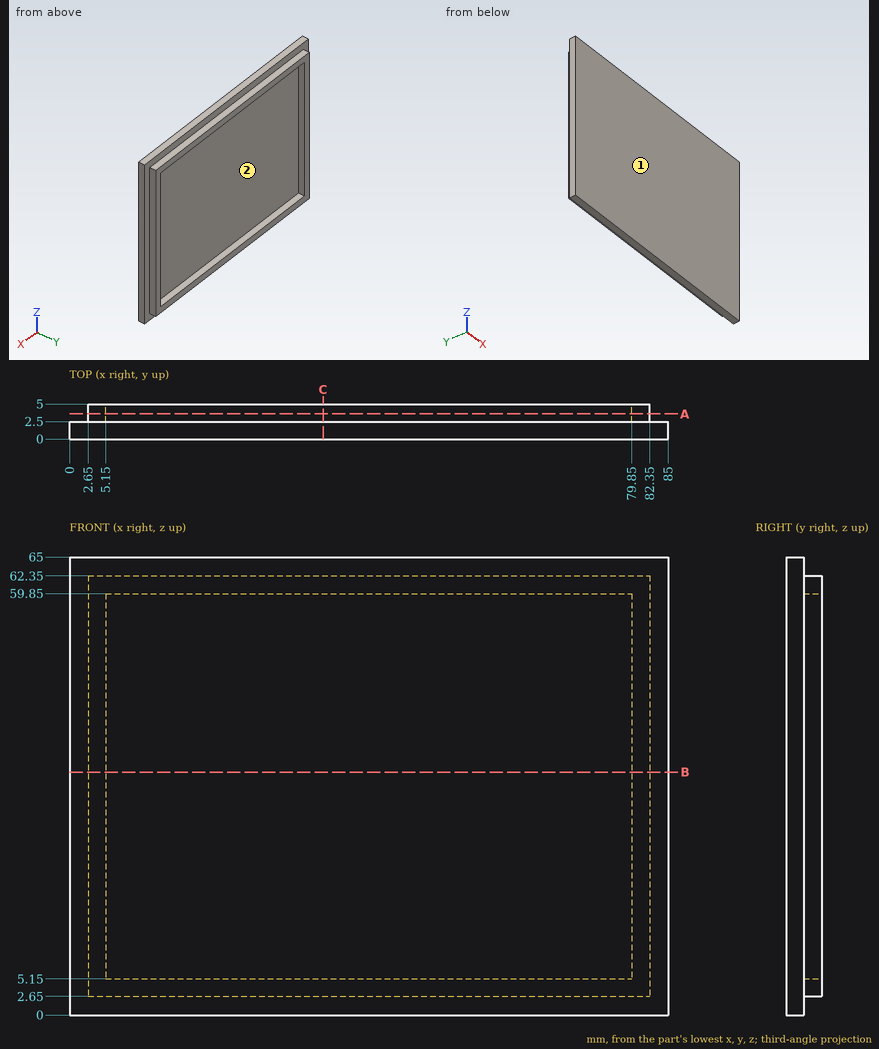
Print and shaded views of the part. All mm, measured from the part's lowest x, y and z. Give positions to 0.01 mm unless a question says otherwise; leave off trailing zeros. Order: outer loops, then holes, each group sorted by start corner. A loop starts at its lowest first (then second) coordinate and runs counter-clockwise, first axis right, second up. Notation, with made-up numbers: (-17.5, -10.75) -> (15.5, -10.75) arc R18 cw to (15.5, 3.25) -> close; hole circle Ø3 at (13.5, -38). An arc over 180 degrees is marked (long way). Use CSV: the item, a comma, the result in double quotes.
1. Band-saw the part on C-C, the plane x = 36. Give the cut face in (y, z).
Outcome:
outline,"(0, 0) -> (2.5, 0) -> (2.5, 2.65) -> (5, 2.65) -> (5, 5.15) -> (2.5, 5.15) -> (2.5, 59.85) -> (5, 59.85) -> (5, 62.35) -> (2.5, 62.35) -> (2.5, 65) -> (0, 65) -> close"
2. Drop flat-ended pins along their axis: pin 1 (2 mm diameter, centred on x = 26, y = 4, fed in from -Z); pin 2 (1.2 mm diameter, centred on x = 27, y = 3.5, fed in from +Z); pin 3 (1.5 mm diameter, centred on x = 44, z = 15.5, fed in from +Y). Give the stop position or say it passes through.
Outcome:
pin 1,"z = 2.65"
pin 2,"z = 62.35"
pin 3,"y = 2.5"
3. Band-saw the part on B-B, the plane z = 34.5. Give the cut face in (x, y).
Outcome:
outline,"(0, 0) -> (85, 0) -> (85, 2.5) -> (82.35, 2.5) -> (82.35, 5) -> (79.85, 5) -> (79.85, 2.5) -> (5.15, 2.5) -> (5.15, 5) -> (2.65, 5) -> (2.65, 2.5) -> (0, 2.5) -> close"
4. Mould opens along Z. For the marked faces 1 and 2 say: +Z half, -Z half, draft (parallel to the pull), parting line (faces both ways), or undercut.
Outcome:
face 1,"draft"
face 2,"undercut"
5. Band-saw the part on A-A, the plane y = 3.6. Give the cut face in (x, z).
Outcome:
outline,"(2.65, 2.65) -> (82.35, 2.65) -> (82.35, 62.35) -> (2.65, 62.35) -> close; hole (5.15, 5.15) -> (79.85, 5.15) -> (79.85, 59.85) -> (5.15, 59.85) -> close"
6. Drill centre lines: line 1 along X through (y, z) = (3.25, 59); line 2 along Z through (x, y) = (67, 3.6); line 3 along Y through (x, z) = (45, 55). Where is each one in solid material? Low to high. Write a range as from..to.
Outcome:
line 1,"2.65..5.15, 79.85..82.35"
line 2,"2.65..5.15, 59.85..62.35"
line 3,"0..2.5"
